```python
from build123d import *

# Parameters (mm, degrees)
SKETCH1_R               = 11
BOSS_EXTRUDE1_DEPTH     = 6.5
CUT_EXTRUDE1_DEPTH      = 17.8597153
CUT_EXTRUDE1_DEPTH_BACK = 17.8597153
SKETCH2_R               = 3
M3_CLEARANCE_HOLE1_D    = 3.9


with BuildPart() as part:
    # Sketch1 → Boss-Extrude1 (new, symmetric)
    with BuildSketch(Plane.XY):
        with Locations(Location((0, 0, 0), (0, 0, 180))):
            Circle(SKETCH1_R)
    extrude(amount=BOSS_EXTRUDE1_DEPTH, both=True)

    # Sketch2 → Cut-Extrude1 (cut, two sides: drawn at the far end of the back side and taken through both)
    with BuildSketch(Plane(origin=(0, 0, 0), x_dir=(1, 0, 0), z_dir=(0, 1, 0)).offset(-CUT_EXTRUDE1_DEPTH_BACK)):
        with Locations(Location((0, 0, 0), (0, 0, 270))):
            Circle(SKETCH2_R)
    extrude(amount=CUT_EXTRUDE1_DEPTH + CUT_EXTRUDE1_DEPTH_BACK, mode=Mode.SUBTRACT)

    # M3 Clearance Hole1 (through all)
    with Locations(Plane.XY.offset(6.5)):
        with Locations((5.656854249, 5.656854249), (-5.656854249, -5.656854249), (-5.656854249, 5.656854249), (5.656854249, -5.656854249)):
            Hole(M3_CLEARANCE_HOLE1_D / 2)


solid = part.part
```
Geometry: final body of the model. Coordinates: model frame, mm. Give positions to 0.01 mm unless a question says otherwise; leave off trailing zeros. Loops run counter-clockwise (first coordinate to the right, second up) from the corner with the lowest first, then second, coordinate; pieces in that order, holes last. Notation, with made-up numbers: (81.25, -3.75) - (116.25, -3.75) arc R32 cw to (116.25, 23.25) - close; hole circle Ø1 at (89.5, 55). An arc over 180 degrees is marked (long way). Answer as CSV lines item,"result". Start each with the question number.
(1) Section query C-C (y = -4.75). Output: boundary loops of the cut face in (x, z), and give its area (3 significant figures).
(2) Ray query, line 1 along X through (y, z) = (6.5, -3.25); line 2 along X through (y, z) = (4.5, -4.75). Return the intervals inside material, ascending. Write a range as [from, to].
(3) Mould query, pull axis Y, two halves, no side actions, for faces 1 (the face through (-7.517, -5.071, -0.091)), 2 (the face through (0, 0, -6.5)), 3 (the face through (-10.492, -3.304, 0.091)). Classes: +Y half, -Y half, draft (parallel to the pull), parting line (faces both ways), or undercut.
(4) Section query A-A (x = 0). Output: boundary loops of the cut face in (y, z).
(5) Section query B-B (z = 0.5). Output: boundary loops of the cut face in (x, y).
(6) Pin query (flat end, axial travel): P1, Ø1.5, axis at y = -8.5, z = -0.5, coming from the +X side; P2, Ø5, axis at x = -5, z = 1.5, coming from the +Y side; P3, Ø5, axis at y = -7, z = 0, coming from the +X side. Return the tip coordinate at first contact, or that it passes through.
(7) Section query D-D (y = 0). Output: boundary loops of the cut face in (x, z).
Worked answers:
1,outline,"(-9.92, -6.5) - (-7.38, -6.5) - (-7.38, 6.5) - (-9.92, 6.5) - close; (-3.93, -6.5) - (3.93, -6.5) - (3.93, 6.5) - (-3.93, 6.5) - close; (7.38, -6.5) - (9.92, -6.5) - (9.92, 6.5) - (7.38, 6.5) - close; hole circle Ø6 at (0, 0)"
1,area,"140 mm^2"
2,line 1,"x = [-8.87, -7.42], [-3.9, 3.9], [7.42, 8.87]"
2,line 2,"x = [-10.04, -7.23], [-4.09, 4.09], [7.23, 10.04]"
3,face 1,"undercut"
3,face 2,"draft"
3,face 3,"parting line"
4,outline,"(-11, -6.5) - (11, -6.5) - (11, -3) - (-11, -3) - close; (-11, 3) - (11, 3) - (11, 6.5) - (-11, 6.5) - close"
5,outline,"(-2.96, -10.59) - (-2.96, 10.59) arc R11 ccw to start; (2.96, -10.59) arc R11 ccw to (2.96, 10.59) - close; hole circle Ø3.9 at (-5.66, -5.66); hole circle Ø3.9 at (-5.66, 5.66); hole circle Ø3.9 at (5.66, -5.66); hole circle Ø3.9 at (5.66, 5.66)"
6,P1,"stops at x = 7.81"
6,P2,"stops at y = 10.71"
6,P3,"stops at x = 10.04"
7,outline,"(-11, -6.5) - (11, -6.5) - (11, 6.5) - (-11, 6.5) - close; hole circle Ø6 at (0, 0)"
